```python
from build123d import *

# Parameters (mm, degrees)
F0_W      = 203.2
F0_H      = 105.2184881944
F1_DEPTH  = 127
F2_T      = -2.54
F4_W      = 24.9819085002
F4_H      = 37.9526205361
F4_W_2    = 151.2214764953
F4_H_2    = 25.4
F5_DEPTH  = 76.2
F6_W      = 148.822195828
F6_H      = 73.4275504947
F7_DEPTH  = 15.24
F9_DEPTH  = 25.4
F10_DEPTH = 33.02


with BuildPart() as f1:
    # F0 (on Top) → F1 (new body)
    with BuildSketch(Plane.XY):
        with Locations((-0.9812270495, 52.6092440972)):
            Rectangle(F0_W, F0_H)
    extrude(amount=F1_DEPTH)

    # F2
    f2_openings = [f1.faces().sort_by_distance(p)[0] for p in [
        (-0.981227, 52.609244, 127),
    ]]
    offset(amount=F2_T, openings=f2_openings)

    # F4 (on face) → F5 (join)
    with BuildSketch(Plane.XZ):
        Polygon((-77.0476683974, 0), (-77.0476683974, 25.4), (-77.1812270495, 25.4), (-77.1812270495, 37.9526205361), (-102.5303602219, 37.9526205361), (-102.5303602219, 0), align=None)
        with Locations((88.0557782948, 18.976310268)):
            Rectangle(F4_W, F4_H)
        with Locations((-0.6120987236, 12.7)):
            Rectangle(F4_W_2, F4_H_2)
    extrude(amount=F5_DEPTH)

    # F6 (on face) → F7 (cut)
    with BuildSketch(Plane.XY.offset(25.4)):
        with Locations((-1.2982971966, -37.2778810561)):
            Rectangle(F6_W, F6_H)
    extrude(amount=-F7_DEPTH, mode=Mode.SUBTRACT)

    # F8 (on face) → F9 (join)
    with BuildSketch(Plane.XY.offset(10.16)):
        Polygon((-50.4458248615, -0.5641058087), (-57.7319078147, -0.5641058087), (-57.7319078147, -44.1493541002), (-59.9848367274, -44.1493541002), (-59.9848367274, -73.9916563034), (-48.2489354908, -73.9916563034), (-48.2489354908, -44.0681837499), (-50.4458248615, -44.0681837499), align=None)
        Polygon((-67.6321908832, -44.1493541002), (-67.6321908832, -0.5641058087), (-75.7093951106, -0.5641058087), (-75.7093951106, -73.9916563034), (-59.9848367274, -73.9916563034), (-59.9848367274, -44.1493541002), align=None)
        Polygon((-30.921860598, -0.5641058087), (-36.0744632781, -0.5641058087), (-36.0744632781, -73.9916563034), (-25.769257918, -73.9916563034), (-26.1848908849, -44.2901365459), (-30.921860598, -44.2901365459), align=None)
        Polygon((-36.0744632781, -0.5641058087), (-40.8624187112, -0.5641058087), (-40.8624187112, -44.0681837499), (-48.2489354908, -44.0681837499), (-48.2489354908, -73.9916563034), (-36.0744632781, -73.9916563034), align=None)
    extrude(amount=F9_DEPTH)

    # F10 (add): faces of the model
    f10_faces = [f1.faces().sort_by_distance(p)[0] for p in [
        (-62.682049349, -22.3567299545, 10.16),
        (-45.6541217864, -22.3161447793, 10.16),
    ]]
    extrude(f10_faces, amount=F10_DEPTH)


solid = f1.part
```
The listing builds one solid part. Answer for the finished solid, in the listing's coordinates (mm). A direction names the side the tool comes from. Give positions to 0.01 mm unless a question says otherwise; leave off trailing zeros. Write each loop counter-clockwise with the first axis right and the second up, starting at its lowest first coordinate (ties: lowest second). Pieces come first, ordered by that corner, then holes. Notation, with made-up numbers: (51, -20.5) -> (57, -20.5) arc R12 ccw to (57, -12.5) -> close; hole circle Ø11 at (84, 39). An arc over 180 degrees is marked (long way). Use one line per item in the form item = value.
1) Section A-A on z = 108 is taken. Write down the section's boundary in (x, y), plus the area to 3 significant figures.
Result:
outline = (-102.58, 0) -> (100.62, 0) -> (100.62, 105.22) -> (-102.58, 105.22) -> close; hole (-100.04, 2.54) -> (98.08, 2.54) -> (98.08, 102.68) -> (-100.04, 102.68) -> close
area = 1,540 mm²
2) Section B-B on y = -32.5 is taken. Write down the section's boundary in (x, z), plus the area to 3 significant figures.
Result:
outline = (-102.53, 0) -> (-77.05, 0) -> (-77.05, 25.4) -> (-77.18, 25.4) -> (-77.18, 37.95) -> (-102.53, 37.95) -> close; (-76.22, 0) -> (75, 0) -> (75, 25.4) -> (73.11, 25.4) -> (73.11, 10.16) -> (-30.92, 10.16) -> (-30.92, 35.56) -> (-40.86, 35.56) -> (-40.86, 43.18) -> (-50.45, 43.18) -> (-50.45, 35.56) -> (-57.73, 35.56) -> (-57.73, 43.18) -> (-67.63, 43.18) -> (-67.63, 35.56) -> (-75.71, 35.56) -> (-75.71, 25.4) -> (-76.22, 25.4) -> close; (75.56, 0) -> (100.55, 0) -> (100.55, 37.95) -> (75.56, 37.95) -> close
area = 4,770 mm²
3) Each of these flat-tipped pins is pushed along its axis until it touches: P1, Ø1, axis at x = 43.5, y = 48.5, coming from the -Z side; P2, Ø5, axis at x = -23, y = -48.5, coming from the +Z side; P3, Ø17, axis at y = -21.5, z = 15.5, coming from the -X side; P4, Ø4, axis at x = 35, z = 77.5, coming from the -Y side. Where does it stop, or does it pass through?
Result:
P1 = 0
P2 = 10.16
P3 = -102.53
P4 = 0
4) For a pull along X with two mould halves and no side action, classify faces 4 (the flat face through (100.547, -38, 19)), 5 (the flat face through (-46, -22, 43.18)), 6 (the flat face through (-51, -37, 35.56)) as +X half, -X half, draft (parallel to the pull), parting line (faces both ways), or undercut.
Result:
face_4 = +X half
face_5 = draft
face_6 = undercut
5) Section C-C on x = -72 is taken. Write down the section's boundary in (y, z), plus the area to 3 significant figures.
Result:
outline = (-76.2, 0) -> (105.22, 0) -> (105.22, 127) -> (102.68, 127) -> (102.68, 2.54) -> (2.54, 2.54) -> (2.54, 127) -> (0, 127) -> (0, 25.4) -> (-0.56, 25.4) -> (-0.56, 35.56) -> (-73.99, 35.56) -> (-73.99, 25.4) -> (-76.2, 25.4) -> close
area = 3,580 mm²
6) Straight lines are drawn through the part: probe 1 along Y at (x, z) = (23.5, 19); probe 2 along X at (y, z) = (-63.5, 7); probe 3 along Y at (x, z) = (46.5, 92). For each, find the intervals that lie inside material, in ascending order.
Result:
probe_1 = -76.2 to -73.99, -0.56 to 2.54, 102.68 to 105.22
probe_2 = -102.53 to -77.05, -76.22 to 75, 75.56 to 100.55
probe_3 = 0 to 2.54, 102.68 to 105.22
7) A tool of negligible diameter and unlimited length cuts with its end or side. For faces 1 (the flat face through (88, -38, 37.953)), 2 (the flat face through (-50.446, -23, 39)), 3 (the flat face through (-29, -44.29, 23)), from which of +Z, -Z, +X, -X, +Y, -Y can it reach the whole face along a straight path? Write none if from no direction.
Result:
face_1 = +Z, +X, -Y
face_2 = +Z, -Y
face_3 = +Z
8) Section D-D on y = 77 is taken. Write down the section's boundary in (x, z).
Result:
outline = (-102.58, 0) -> (100.62, 0) -> (100.62, 127) -> (98.08, 127) -> (98.08, 2.54) -> (-100.04, 2.54) -> (-100.04, 127) -> (-102.58, 127) -> close
